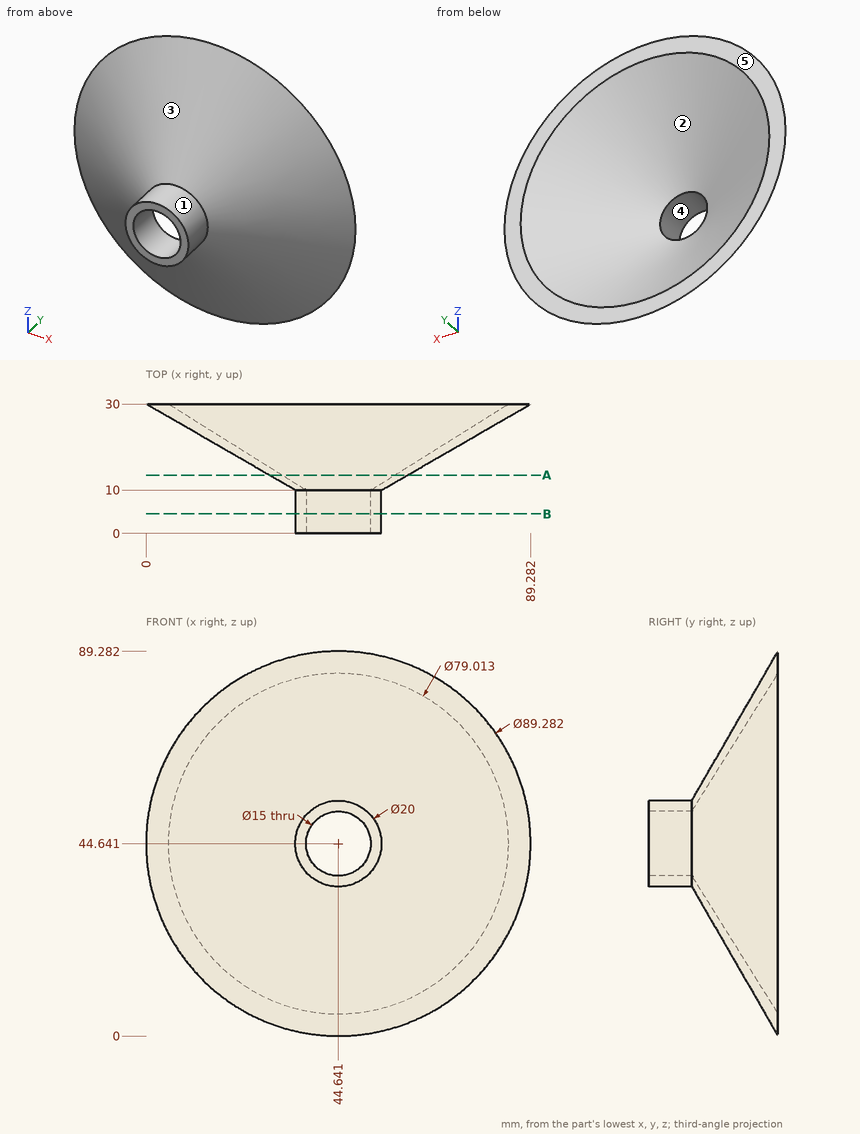
Here's the drawing with two shaded views (mm, measured from the low corner). I have some questions. A direction names the side the tool comes from. Coordinates: 2 decimals unless noted, no trailing zeros. Loops run counter-clockwise (first coordinate to the right, second up) from the corner with the lowest first, then second, coordinate; pieces in that order, holes last. Notation, with made-up numbers: (87, 9.25) -> (145, 9.25) arc R14 ccw to (145, 30.25) -> close; hole circle Ø7 at (-2.5, 75). An arc over 180 degrees is marked (long way). Put each result on its own line as item: value. Start each with the question number.
Q1. I want a section at B-B (y = 4.5). Write out the boundary of the cut face in (x, z).
Q2. I'm going to push flat-ended pins straight in: P1, Ø4, axis at x = 30, z = 25.5, coming from the -Y side (1 decimal); P2, Ø8, axis at x = 38.5, y = 6.5, coming from the +Z side; P3, Ø6, axis at x = 40.5, z = 52.5, coming from the +Y side; P4, Ø9, axis at x = 44.64, z = 44.64, coming from the +Y side. Where does each tip first touch, or does it pass through?
Q3. I want a section at A-A (y = 13.5). Write out the boundary of the cut face in (x, z) (1 decimal), plus the area to 3 significant figures.
Q4. If I drill on line 1 (X direction, y = 1.5, z = 44.5); line 2 (Z direction, x = 38, y = 22) (1 decimal); line 3 (Z direction, x = 27.5, y = 20) (1 decimal), over which ranges is the centre line in solid material (lowest first)? Write a range as [from, to].
Q5. For the marked faces 1 and 2, which set-ups out of +Z, -Z, +X, -X, +Y, -Y let a thin tool reach every point of the face, with its end or its side?
Q6. Thinking about a two-plate mould opening in Z: for the marked faces 3, 4 and 5, which applies, pulls with the +Z half, pulls with the -Z half, needs draft (parallel to the pull), parting line crosses it, or undercut?
Taken from the geometry:
1. outline: circle Ø20 at (44.64, 44.64); hole circle Ø15 at (44.64, 44.64)
2. P1: stops at y = 17
2. P2: stops at z = 54.41
2. P3: stops at y = 12.74
2. P4: passes through
3. outline: circle Ø32.1 at (44.6, 44.6); hole circle Ø26.2 at (44.6, 44.6)
3. area: 271 mm2
4. line 1: x = [34.64, 37.14], [52.14, 54.64]
4. line 2: z = [14.6, 18.8], [70.5, 74.7]
4. line 3: z = [23.4, 28.6], [60.7, 65.9]
5. face 1: -Y
5. face 2: +Y
6. face 3: parting line crosses it
6. face 4: undercut
6. face 5: needs draft
